Design review of the part built by this model. Coordinates are the model's own, in mm. Face numbers are marked on the shaded views. A direction names the side the tool comes from. Give positions to 0.01 mm unless a question says otherwise; leave off trailing zeros. Order: outer loops, then holes, each group sorted by start corner. A loop starts at its lowest first (then second) coordinate and runs counter-clockwise, first axis right, second up.
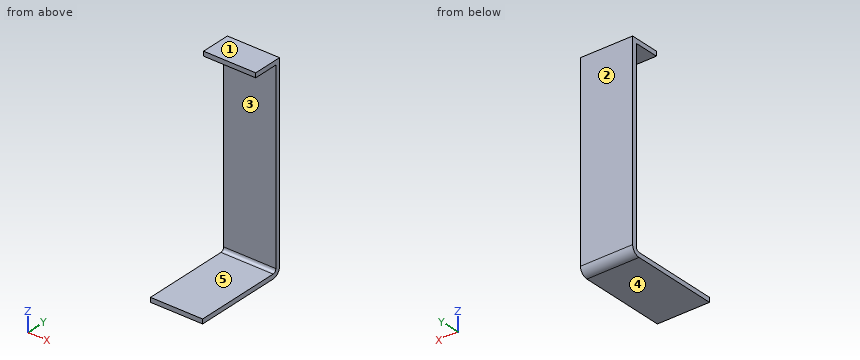
```python
from build123d import *

# Parameters (mm, degrees)
SKETCH1_W           = 23
SKETCH1_H           = 87
BOSS_EXTRUDE1_DEPTH = 42
FILLET1_R           = 3.5
CUT_EXTRUDE1_DEPTH  = 24
SKETCH3_W           = 2
SKETCH3_H           = 40
CUT_EXTRUDE3_DEPTH  = 24
SKETCH4_W           = 83
SKETCH4_H           = 2
CUT_EXTRUDE5_DEPTH  = 24
SKETCH6_W           = 23
SKETCH6_H           = 2
BOSS_EXTRUDE2_DEPTH = 11


with BuildPart() as part:
    # Sketch1 → Boss-Extrude1 (new body)
    with BuildSketch(Plane(origin=(0, 0, 0), x_dir=(1, 0, 0), z_dir=(0, 1, 0))):
        with Locations((14.807125307, -11.663390663)):
            Rectangle(SKETCH1_W, SKETCH1_H)
    extrude(amount=BOSS_EXTRUDE1_DEPTH)

    # Fillet1
    fillet1_edges = [part.edges().sort_by_distance(p)[0] for p in [
        (14.807125307, 42, -31.836609337),
    ]]
    fillet(fillet1_edges, radius=FILLET1_R)

    # Sketch2 → Cut-Extrude1 (cut, through all)
    with BuildSketch(Plane(origin=(26.307125307, 0, 0), x_dir=(0, 0, -1), z_dir=(1, 0, 0))):
        with BuildLine():
            Line((29.836609337, 2), (29.836609337, 38.5))
            ThreePointArc((29.836609337, 38.5), (29.397269508, 39.560660172), (28.336609337, 40))
            Line((28.336609337, 40), (-53.163390663, 40))
            Line((-53.163390663, 40), (-53.163390663, 2))
            Line((-53.163390663, 2), (29.836609337, 2))
        make_face()
    extrude(amount=-CUT_EXTRUDE1_DEPTH, mode=Mode.SUBTRACT)

    # Sketch3 → Cut-Extrude3 (cut, through all)
    with BuildSketch(Plane(origin=(26.307125307, 0, 0), x_dir=(0, 0, -1), z_dir=(1, 0, 0))):
        with Locations((-54.163390663, 20)):
            Rectangle(SKETCH3_W, SKETCH3_H)
    extrude(amount=-CUT_EXTRUDE3_DEPTH, mode=Mode.SUBTRACT)

    # Sketch4 → Cut-Extrude5 (cut, through all)
    with BuildSketch(Plane(origin=(26.307125307, 0, 0), x_dir=(0, 0, -1), z_dir=(1, 0, 0))):
        with Locations((-11.663390663, 1)):
            Rectangle(SKETCH4_W, SKETCH4_H)
    extrude(amount=-CUT_EXTRUDE5_DEPTH, mode=Mode.SUBTRACT)

    # Sketch6 → Boss-Extrude2 (add)
    with BuildSketch(Plane.XZ.offset(-40)):
        with Locations((14.807125307, 54.163390663)):
            Rectangle(SKETCH6_W, SKETCH6_H)
    extrude(amount=BOSS_EXTRUDE2_DEPTH)


solid = part.part
```
1. Take a section at B-B (x = 22.25). State the section outline as (y, z) points.
Recorded:
outline: (0, -31.84) - (38.5, -31.84) arc R3.5 ccw to (42, -28.34) - (42, 55.16) - (29, 55.16) - (29, 53.16) - (40, 53.16) - (40, -28.34) arc R1.5 cw to (38.5, -29.84) - (0, -29.84) - close
2. Take a section at D-D (z = -24). State the section outline as (x, y) points, then the cut area to 3 significant figures.
Recorded:
outline: (3.31, 40) - (26.31, 40) - (26.31, 42) - (3.31, 42) - close
area: 46.0 mm2
3. Draft analysis for pull direction Z (two halves, no side actions). For the marked faces 1, 2 and 3, state which applies: pulls with the +Z half, pulls with the -Z half, needs draft (parallel to the pull), parting line crosses it, or undercut.
Recorded:
face 1: pulls with the +Z half
face 2: needs draft
face 3: undercut
4. Machinability: for the marked faces 4 and 5, which of the approach directions +Z, -Z, +X, -X, +Y, -Y give a long, thin tool a straight path to every point of the face, cutting with its end or side? Answer none if there is none.
Recorded:
face 4: -Z, +X, -X, +Y, -Y
face 5: +X, -X, -Y
5. For pin 1 (7 mm diameter, centred on x = 20.5, z = -5, fed in from -Y); pin 2 (5 mm diameter, centred on x = 16.5, y = 15.5, fed in from +Z); pin 3 (0.6 mm diameter, centred on x = 10.5, z = 53.5, fed in from -Y), all flat-tipped, find the tip position at first contact; note any pin that passes through.
Recorded:
pin 1: stops at y = 40
pin 2: stops at z = -29.84
pin 3: stops at y = 29
6. For line 1 along Z through (x, y) = (18.25, 29.5); line 2 along Y through (x, z) = (22, -13.5); line 3 along Z through (x, y) = (5.5, 10.5), list the stretches that pass through material, from the lowest coordinate up.
Recorded:
line 1: z = -31.84 to -29.84, 53.16 to 55.16
line 2: y = 40 to 42
line 3: z = -31.84 to -29.84
7. Take a section at C-C (y = 23.5). State the section outline as (x, z) points.
Recorded:
outline: (3.31, -31.84) - (26.31, -31.84) - (26.31, -29.84) - (3.31, -29.84) - close
8. Take a section at A-A (y = 33). State the section outline as (x, z) points, then the cut area to 3 significant figures.
Recorded:
outline: (3.31, -31.84) - (26.31, -31.84) - (26.31, -29.84) - (3.31, -29.84) - close; (3.31, 53.16) - (26.31, 53.16) - (26.31, 55.16) - (3.31, 55.16) - close
area: 92.0 mm2
